The listing builds one solid part. Answer for the finished solid, in the listing's coordinates (mm). Face numbers are marked on the shaded views. A direction names the side the tool comes from. Coordinates: 2 decimals unless noted, no trailing zeros. Order: outer loops, then holes, each group sorted by start corner. A loop starts at its lowest first (then second) coordinate and runs counter-clockwise, first axis right, second up. Notation, with made-up numbers: (77, 86.5) -> (91, 86.5) arc R22 ccw to (91, 108.5) -> close; hole circle Ø10 at (-5, 69). An arc over 180 degrees is marked (long way). Return JSON: item names as keys, results as strings.
```python
from build123d import *

# Parameters (mm, degrees)
F0_R     = 1.524
F0_R_2   = 1.27
F0_W     = 5.08
F0_H     = 26.162
F1_DEPTH = 3.81
F2_R     = 1.90499
F3_R     = 1.016
F4_DEPTH = 3.81
F5_R     = 2.794
F6_DEPTH = 2.54


# Not quite as in the source:
# - a fillet or chamfer is up to 0.001 mm smaller than in the source, because OpenCascade refuses the exact size


with BuildPart() as f1:
    # F0 (on Top) → F1 (new body)
    with BuildSketch(Plane.XY):
        with BuildLine():
            ThreePointArc((-8.89, 31.75), (-11.43, 29.21), (-8.89, 26.67))
            Line((-8.89, 26.67), (-4.064, 26.67))
            Line((-4.064, 26.67), (-4.064, -1.524))
            Line((-4.064, -1.524), (-7.874, -1.524))
            Line((-7.874, -1.524), (-7.874, -13.97))
            Line((-7.874, -13.97), (-8.89, -13.97))
            ThreePointArc((-8.89, -13.97), (-10.6860512242, -18.3060512242), (-6.35, -16.51))
            Line((-6.35, -16.51), (-6.35, -4.064))
            Line((-6.35, -4.064), (6.35, -4.064))
            Line((6.35, -4.064), (6.35, -16.51))
            ThreePointArc((6.35, -16.51), (10.6860512242, -18.3060512242), (8.89, -13.97))
            Line((8.89, -13.97), (7.874, -13.97))
            Line((7.874, -13.97), (7.874, -1.524))
            Line((7.874, -1.524), (4.064, -1.524))
            Line((4.064, -1.524), (4.064, 26.67))
            Line((4.064, 26.67), (8.89, 26.67))
            ThreePointArc((8.89, 26.67), (11.43, 29.21), (8.89, 31.75))
            Line((8.89, 31.75), (-8.89, 31.75))
        make_face()
        Circle(F0_R, mode=Mode.SUBTRACT)
        with Locations((-8.89, 29.21)):
            Circle(F0_R_2, mode=Mode.SUBTRACT)
        with Locations((0, 17.145)):
            Rectangle(F0_W, F0_H, mode=Mode.SUBTRACT)
        with Locations((8.89, 29.21)):
            Circle(F0_R_2, mode=Mode.SUBTRACT)
    extrude(amount=F1_DEPTH)

    # F2 (radius 1.905 in the source; OpenCascade refuses exactly that, so slightly less here)
    f2_edges = [f1.edges().sort_by_distance(p)[0] for p in [
        (6.35, -4.064, 1.905),
        (-6.35, -4.064, 1.905),
        (-4.064, -1.524, 1.905),
        (-7.874, -1.524, 1.905),
        (7.874, -1.524, 1.905),
        (4.064, 26.67, 1.905),
        (4.064, -1.524, 1.905),
        (-4.064, 26.67, 1.905),
        (2.54, 30.226, 1.905),
        (-2.54, 30.226, 1.905),
        (-2.54, 4.064, 1.905),
        (2.54, 4.064, 1.905),
        (7.874, -13.97, 1.905),
        (-7.874, -13.97, 1.905),
    ]]
    fillet(f2_edges, radius=F2_R)

    # F3 (on face) → F4 (join)
    with BuildSketch(Plane.XY.offset(3.81)):
        with Locations((-8.89, -16.51)):
            Circle(F3_R)
        with Locations((8.89, -16.51)):
            Circle(F3_R)
    extrude(amount=F4_DEPTH)

    # F5 (on face) → F6 (cut)
    with BuildSketch(Plane.XY.offset(3.81)):
        Circle(F5_R)
    extrude(amount=-F6_DEPTH, mode=Mode.SUBTRACT)


solid = f1.part
```
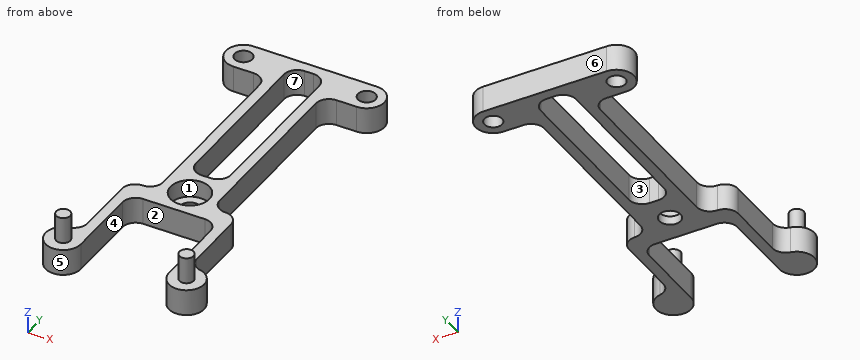
Item 1: The part is cut by section C-C on y = 29.21. Determine the outline of the cut face in (x, z).
Answer list:
{"outline": "(-11.43, 0) -> (-10.16, 0) -> (-10.16, 3.81) -> (-11.43, 3.81) -> close; (-7.62, 0) -> (-2.32, 0) -> (-2.32, 3.81) -> (-7.62, 3.81) -> close; (2.32, 0) -> (7.62, 0) -> (7.62, 3.81) -> (2.32, 3.81) -> close; (10.16, 0) -> (11.43, 0) -> (11.43, 3.81) -> (10.16, 3.81) -> close"}
Item 2: The part is cut by section B-B on y = 19.5. Determine the outline of the cut face in (x, z), plus the area to 3 significant figures.
Answer list:
{"outline": "(-4.06, 0) -> (-2.54, 0) -> (-2.54, 3.81) -> (-4.06, 3.81) -> close; (2.54, 0) -> (4.06, 0) -> (4.06, 3.81) -> (2.54, 3.81) -> close", "area": "11.6 mm2"}
Item 3: Find the intervals of material crossed by probe 1 along Y at (x, z) = (0, 2.25); probe 2 along Y at (x, z) = (8.89, 1.3); probe 3 along X at (y, z) = (11.5, 3.25), in increasing order.
Answer list:
{"probe 1": "-4.06 to -2.79, 2.79 to 4.06, 30.23 to 31.75", "probe 2": "-19.05 to -13.84, 26.67 to 27.94, 30.48 to 31.75", "probe 3": "-4.06 to -2.54, 2.54 to 4.06"}
Item 4: Which of the six approach directions +Z, -Z, +X, -X, +Y, -Y give full straight-line access (tool end or side, diameter ignored) to the marked faces 1, 2 and 3?
Answer list:
{"face 1": "+Z", "face 2": "+Z, -Z, -Y", "face 3": "+Z, -Z"}
Item 5: Determine the mould class of the marked faces 4, 5, 6 and 7 for opening direction Y: pulls with the +Y half, pulls with the -Y half, needs draft (parallel to the pull), parting line crosses it, or undercut.
Answer list:
{"face 4": "needs draft", "face 5": "undercut", "face 6": "pulls with the +Y half", "face 7": "undercut"}
Item 6: Flat-ended cylindrical pins translate along their axes: pin 1 (0.9 mm diameter, centred on x = 6.5, z = 2, fed in from -Y); pin 2 (4 mm diameter, centred on x = 0.5, z = 2.5, fed in from -Y); pin 3 (5 mm diameter, centred on x = -6, y = 23.5, fed in from -Z); pin 4 (1.5 mm diameter, centred on y = 20, z = 4.5, fed in from +X). Find the tip coordinate at first contact, or state that the pin passes through.
Answer list:
{"pin 1": "y = -18.15", "pin 2": "y = -4.06", "pin 3": "z = 0", "pin 4": "x = 4.06"}
Item 7: The part is cut by section A-A on x = 0. Determine the outline of the cut face in (y, z), plus the area to 3 significant figures.
Answer list:
{"outline": "(-4.06, 0) -> (-1.52, 0) -> (-1.52, 1.27) -> (-2.79, 1.27) -> (-2.79, 3.81) -> (-4.06, 3.81) -> close; (1.52, 0) -> (4.06, 0) -> (4.06, 3.81) -> (2.79, 3.81) -> (2.79, 1.27) -> (1.52, 1.27) -> close; (30.23, 0) -> (31.75, 0) -> (31.75, 3.81) -> (30.23, 3.81) -> close", "area": "18.7 mm2"}
Item 8: The part is cut by section D-D on z = 7. Determine the outline of the cut face in (x, y).
Answer list:
{"outline": "circle Ø2.03 at (-8.89, -16.51); circle Ø2.03 at (8.89, -16.51)"}
